from build123d import *

# Parameters (mm, degrees)
BOSS_EXTRUDE1_DEPTH = 12.7
SKETCH2_W           = 12.7
SKETCH2_H           = 63.5
BOSS_EXTRUDE2_DEPTH = 31.75
SKETCH3_W           = 18
SKETCH3_H           = 3
CUT_EXTRUDE1_DEPTH  = 19.05
SKETCH4_R           = 2
CUT_EXTRUDE2_DEPTH  = 59.973007597
SKETCH5_R           = 2
CUT_EXTRUDE3_DEPTH  = 64.181702256
SKETCH6_W           = 63.5
SKETCH6_H           = 12.7
CUT_EXTRUDE4_DEPTH  = 11.05
SKETCH7_W           = 12.7
SKETCH7_H           = 63.5
CUT_EXTRUDE5_DEPTH  = 11.05
BOSS_EXTRUDE3_START = 3.175
SKETCH8_W           = 33.4
SKETCH8_H           = 63.5
SKETCH8_R           = 2
SKETCH8_W_2         = 6
SKETCH8_H_2         = 18
BOSS_EXTRUDE3_DEPTH = 3.175
SKETCH9_R           = 1.25
CUT_EXTRUDE6_DEPTH  = 12.7


with BuildPart() as part:
    # Sketch1 → Boss-Extrude1 (new body)
    with BuildSketch(Plane(origin=(0, 0, 0), x_dir=(1, 0, 0), z_dir=(0, 1, 0))):
        Polygon((-22.225, 31.75), (-22.225, -31.75), (0, -31.75), (0, -24.875), (-3, -24.875), (-3, -6.875), (0, -6.875), (0, 0), (0, 6.875), (-3, 6.875), (-3, 24.875), (0, 24.875), (0, 31.75), align=None)
        Polygon((0, -24.875), (0, -31.75), (22.225, -31.75), (22.225, 31.75), (0, 31.75), (0, 24.875), (3, 24.875), (3, 6.875), (0, 6.875), (0, 0), (0, -6.875), (3, -6.875), (3, -24.875), align=None)
    extrude(amount=BOSS_EXTRUDE1_DEPTH)

    # Sketch2 → Boss-Extrude2 (add)
    with BuildSketch(Plane.XZ):
        with Locations((-15.875, 0)):
            Rectangle(SKETCH2_W, SKETCH2_H)
    extrude(amount=BOSS_EXTRUDE2_DEPTH)

    # Sketch3 → Cut-Extrude1 (cut)
    with BuildSketch(Plane.ZY.offset(22.225)):
        with Locations((-15.875, -8.025)):
            Rectangle(SKETCH3_W, SKETCH3_H)
        with Locations((-15.875, -11.025)):
            Rectangle(SKETCH3_W, SKETCH3_H)
        with Locations((15.875, -8.025)):
            Rectangle(SKETCH3_W, SKETCH3_H)
        with Locations((15.875, -11.025)):
            Rectangle(SKETCH3_W, SKETCH3_H)
    extrude(amount=-CUT_EXTRUDE1_DEPTH, mode=Mode.SUBTRACT)

    # Sketch4 → Cut-Extrude2 (cut, through all)
    with BuildSketch(Plane(origin=(0, 12.7, 0), x_dir=(1, 0, 0), z_dir=(0, 1, 0))):
        with Locations(Location((-15.875, 15.875, 0), (0, 0, 270))):
            Circle(SKETCH4_R)
        with Locations(Location((-15.875, -15.875, 0), (0, 0, 270))):
            Circle(SKETCH4_R)
    extrude(amount=-CUT_EXTRUDE2_DEPTH, mode=Mode.SUBTRACT)

    # Sketch5 → Cut-Extrude3 (cut, through all)
    with BuildSketch(Plane.ZY.offset(22.225)):
        with Locations((-15.875, 6.35)):
            Circle(SKETCH5_R)
        with Locations((15.875, 6.35)):
            Circle(SKETCH5_R)
    extrude(amount=-CUT_EXTRUDE3_DEPTH, mode=Mode.SUBTRACT)

    # Sketch6 → Cut-Extrude4 (cut)
    with BuildSketch(Plane(origin=(22.225, 0, 0), x_dir=(0, 0, -1), z_dir=(1, 0, 0))):
        with Locations((0, 6.35)):
            Rectangle(SKETCH6_W, SKETCH6_H)
    extrude(amount=-CUT_EXTRUDE4_DEPTH, mode=Mode.SUBTRACT)

    # Sketch7 → Cut-Extrude5 (cut)
    with BuildSketch(Plane.XZ.offset(31.75)):
        with Locations((-15.875, 0)):
            Rectangle(SKETCH7_W, SKETCH7_H)
    extrude(amount=-CUT_EXTRUDE5_DEPTH, mode=Mode.SUBTRACT)

    # Sketch8 → Boss-Extrude3 (add)
    with BuildSketch(Plane(origin=(0, 12.7, 0), x_dir=(1, 0, 0), z_dir=(0, 1, 0)).offset(BOSS_EXTRUDE3_START)):
        with Locations((-5.525, 0)):
            Rectangle(SKETCH8_W, SKETCH8_H)
        with Locations(Location((-15.875, 15.875, 0), (0, 0, 90))):
            Circle(SKETCH8_R, mode=Mode.SUBTRACT)
        with Locations(Location((-15.875, -15.875, 0), (0, 0, 90))):
            Circle(SKETCH8_R, mode=Mode.SUBTRACT)
        with Locations((0, -15.875)):
            Rectangle(SKETCH8_W_2, SKETCH8_H_2, mode=Mode.SUBTRACT)
        with Locations((0, 15.875)):
            Rectangle(SKETCH8_W_2, SKETCH8_H_2, mode=Mode.SUBTRACT)
    extrude(amount=-BOSS_EXTRUDE3_DEPTH)

    # Sketch9 → Cut-Extrude6 (cut)
    with BuildSketch(Plane(origin=(0, 15.875, 0), x_dir=(1, 0, 0), z_dir=(0, 1, 0))):
        with Locations(Location((-15.875, 26.75, 0), (0, 0, 270))):
            Circle(SKETCH9_R)
        with Locations(Location((-15.875, -26.75, 0), (0, 0, 270))):
            Circle(SKETCH9_R)
        with Locations(Location((6.35, 26.75, 0), (0, 0, 270))):
            Circle(SKETCH9_R)
        with Locations(Location((6.35, -26.75, 0), (0, 0, 270))):
            Circle(SKETCH9_R)
    extrude(amount=-CUT_EXTRUDE6_DEPTH, mode=Mode.SUBTRACT)


solid = part.part
Could you check a few things on this model? Use its own coordinates, in mm. A direction names the side the tool comes from. Give positions to 0.01 mm unless a question says otherwise; leave off trailing zeros. Order: outer loops, then holes, each group sorted by start corner. A loop starts at its lowest first (then second) coordinate and runs counter-clockwise, first axis right, second up. Notation, with made-up numbers: (56.25, 48.25) - (66.25, 48.25) arc R11 cw to (66.25, 58.25) - close; hole circle Ø3 at (0.5, 62). An arc over 180 degrees is marked (long way). Return JSON: item names as keys, results as strings. Group by question number.
Q1. Will these pins go through, and if not, where does the flat tip stop? pin 1 Ø12 at (x, z) = (7.5, -4) entering from -Y; pin 2 Ø2.5 at (y, z) = (6.35, 15.875) entering from +X.
Q2. Suppose I cut it at A-A, the plane x = -11.5. Please give me the cut outline in (y, z) (3 decimals), and give its area (3 significant figures).
Q3. Suppose I cut it at D-D, the plane x = 6.35. Please give me the cut outline in (y, z) (3 decimals), and give its area (3 significant figures).
Q4. Suppose I cut it at B-B, the plane y = -10.5. Please give me the cut outline in (x, z) (3 decimals).
Q5. Which directions (+Z, -Z, +X, -X, +Y, -Y) give clear straight access to the entire face, cutting with the end or side of a thin tool? Please do faces 5 (the face through (-22.225, -2, 0)), 6 (the face through (-9.525, -10, 0)), 7 (the face through (-16, -9, -24.875)), 8 (the face through (-3, 10, -16)), 9 (the face through (-14.82, 9.61, -26.08)).
Q6. Thinking about a two-plate mould opening in Y: for faces 1 (the face through (-17, -12.525, -18)), 2 (the face through (3, 10, -16)), 3 (the face through (-16, -20.7, 0)), 4 (the face through (-16, 3.175, -27)), which applies, pulls with the +Y half, pulls with the -Y half, needs draft (parallel to the pull), parting line crosses it, or undercut?
Q7. Suppose I cut it at C-C, the plane z = 26.75. Please give me the cut outline in (x, y) (3 decimals), and give its area (3 significant figures).
Q8. Please list where these lines run through material, in increasing order: line 1 along Z through (x, y) = (-19, 6.35) (3 decimals); line 2 along X through (y, z) = (10, -26.75) (3 decimals); line 3 along Z through (x, y) = (-1, 2) (3 decimals). Write a range as [from, to].
Resolved:
{
 "1": {"pin 1": "stops at y = 0", "pin 2": "passes through"},
 "2": {"outline": "(-20.7, -31.75) - (15.875, -31.75) - (15.875, 31.75) - (-20.7, 31.75) - close; hole (-12.525, -24.875) - (-6.525, -24.875) - (-6.525, -6.875) - (-12.525, -6.875) - close; hole (-12.525, 6.875) - (-6.525, 6.875) - (-6.525, 24.875) - (-12.525, 24.875) - close; hole circle Ø4 at (6.35, -15.875); hole circle Ø4 at (6.35, 15.875)", "area": "2,080 mm2"},
 "3": {"outline": "(0, -31.75) - (15.875, -31.75) - (15.875, -28) - (3.175, -28) - (3.175, -25.5) - (15.875, -25.5) - (15.875, 25.5) - (3.175, 25.5) - (3.175, 28) - (15.875, 28) - (15.875, 31.75) - (0, 31.75) - close; hole circle Ø4 at (6.35, -15.875); hole circle Ø4 at (6.35, 15.875)", "area": "919 mm2"},
 "4": {"outline": "(-22.225, -31.75) - (-9.525, -31.75) - (-9.525, -24.875) - (-22.225, -24.875) - close; (-22.225, -6.875) - (-9.525, -6.875) - (-9.525, 6.875) - (-22.225, 6.875) - close; (-22.225, 24.875) - (-9.525, 24.875) - (-9.525, 31.75) - (-22.225, 31.75) - close"},
 "5": {"face 5": "+Z, -Z, -X, +Y, -Y", "face 6": "+Z, -Z, +X, -Y", "face 7": "+X, -X", "face 8": "+Y, -Y", "face 9": "+Y"},
 "6": {"face 1": "undercut", "face 2": "needs draft", "face 3": "pulls with the -Y half", "face 4": "pulls with the +Y half"},
 "7": {"outline": "(-22.225, -20.7) - (-9.525, -20.7) - (-9.525, 0) - (11.175, 0) - (11.175, 15.875) - (7.6, 15.875) - (7.6, 3.175) - (5.1, 3.175) - (5.1, 15.875) - (-14.625, 15.875) - (-14.625, 3.175) - (-17.125, 3.175) - (-17.125, 15.875) - (-22.225, 15.875) - close", "area": "730 mm2"},
 "8": {"line 1": "z = [-31.75, -17.875], [-13.875, 13.875], [17.875, 31.75]", "line 2": "x = [-22.225, -17.125], [-14.625, 5.1], [7.6, 11.175]", "line 3": "z = [-31.75, -24.875], [-6.875, 6.875], [24.875, 31.75]"}
}
